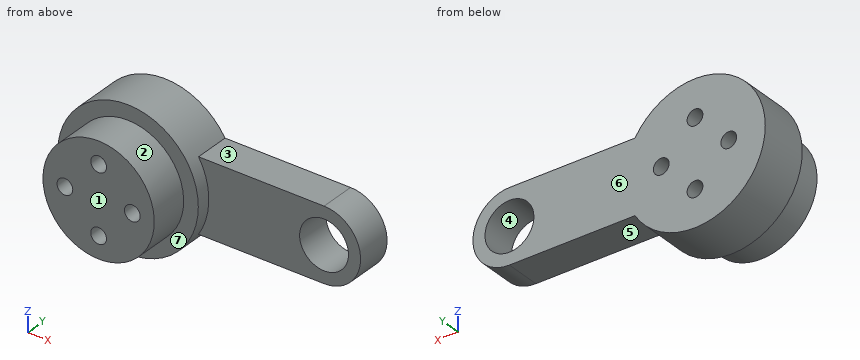
```python
from build123d import *

# Parameters (mm, degrees)
SKETCH_1_R      = 9.9
SKETCH_1_R_2    = 1.4
EXTRUDE_1_DEPTH = 7
SKETCH_2_R      = 12.5
SKETCH_2_R_2    = 1.4
EXTRUDE_2_DEPTH = 2.5
SKETCH_3_R      = 1.4
SKETCH_3_R_2    = 4.35
EXTRUDE_3_DEPTH = 6.3


with BuildPart() as part:
    # 草图1 → 凸台-拉伸1 (new body)
    with BuildSketch(Plane(origin=(0, 0, 0), x_dir=(1, 0, 0), z_dir=(0, 1, 0))):
        with Locations(Location((0, 0, 0), (0, 0, 270))):
            Circle(SKETCH_1_R)
        with Locations(Location((6, 0, 0), (0, 0, 270))):
            Circle(SKETCH_1_R_2, mode=Mode.SUBTRACT)
        with Locations(Location((0, -6, 0), (0, 0, 270))):
            Circle(SKETCH_1_R_2, mode=Mode.SUBTRACT)
        with Locations(Location((-6, 0, 0), (0, 0, 270))):
            Circle(SKETCH_1_R_2, mode=Mode.SUBTRACT)
        with Locations(Location((0, 6, 0), (0, 0, 270))):
            Circle(SKETCH_1_R_2, mode=Mode.SUBTRACT)
    extrude(amount=EXTRUDE_1_DEPTH)

    # 草图2 → 凸台-拉伸2 (add)
    with BuildSketch(Plane(origin=(0, 7, 0), x_dir=(1, 0, 0), z_dir=(0, 1, 0))):
        with Locations(Location((0, 0, 0), (0, 0, 270))):
            Circle(SKETCH_2_R)
        with Locations(Location((-6, 0, 0), (0, 0, 270))):
            Circle(SKETCH_2_R_2, mode=Mode.SUBTRACT)
        with Locations(Location((0, -6, 0), (0, 0, 270))):
            Circle(SKETCH_2_R_2, mode=Mode.SUBTRACT)
        with Locations(Location((6, 0, 0), (0, 0, 270))):
            Circle(SKETCH_2_R_2, mode=Mode.SUBTRACT)
        with Locations(Location((0, 6, 0), (0, 0, 270))):
            Circle(SKETCH_2_R_2, mode=Mode.SUBTRACT)
    extrude(amount=EXTRUDE_2_DEPTH)

    # 草图3 → 凸台-拉伸3 (add)
    with BuildSketch(Plane(origin=(0, 9.5, 0), x_dir=(1, 0, 0), z_dir=(0, 1, 0))):
        with BuildLine():
            Line((33, 6.5), (10.677078252, 6.5))
            ThreePointArc((10.677078252, 6.5), (-12.5, 0), (10.677078252, -6.5))
            Line((10.677078252, -6.5), (33, -6.5))
            ThreePointArc((33, -6.5), (39.5, 0), (33, 6.5))
        make_face()
        with Locations(Location((6, 0, 0), (0, 0, 270))):
            Circle(SKETCH_3_R, mode=Mode.SUBTRACT)
        with Locations(Location((-6, 0, 0), (0, 0, 270))):
            Circle(SKETCH_3_R, mode=Mode.SUBTRACT)
        with Locations(Location((33, 0, 0), (0, 0, 270))):
            Circle(SKETCH_3_R_2, mode=Mode.SUBTRACT)
        with Locations(Location((0, 6, 0), (0, 0, 270))):
            Circle(SKETCH_3_R, mode=Mode.SUBTRACT)
        with Locations(Location((0, -6, 0), (0, 0, 270))):
            Circle(SKETCH_3_R, mode=Mode.SUBTRACT)
    extrude(amount=EXTRUDE_3_DEPTH)


solid = part.part
```
The listing builds one solid part. Answer for the finished solid, in the listing's coordinates (mm). Face numbers are marked on the shaded views. A direction names the side the tool comes from. Coordinates: 2 decimals unless noted, no trailing zeros. Write each loop counter-clockwise with the first axis right and the second up, starting at its lowest first coordinate (ties: lowest second). Pieces come first, ordered by that corner, then holes. Notation, with made-up numbers: (78, -27.75) - (83, -27.75) arc R9 cw to (83, -11.75) - close; hole circle Ø10 at (25.5, -6). An arc over 180 degrees is marked (long way). Return JSON: item names as keys, results as strings. Group by question number.
Q1. For a pull along Z with two mould halves and no side action, classify the marked faces 1, 2, 3 and 4 as +Z half, -Z half, draft (parallel to the pull), parting line (faces both ways), or undercut.
Q2. Find the intervals of material crossed by line 1 along X through (y, z) = (13, 0); line 2 along X through (y, z) = (14.75, 1); line 3 along X through (y, z) = (11.5, -6), in increasing order. Write a range as [from, to].
Q3. The part is cut by section D-D on x = 32. Write down the section's boundary in (y, z), and give its area (3 significant figures).
Q4. The part is cut by section A-A on z = 0. Write down the section's boundary in (x, y).
Q5. The part is cut by section B-B on y = 12.25. Write down the section's boundary in (x, z), and give its area (3 significant figures).
Q6. Flat-ended cylindrical pins translate along their axes: pin 1 Ø5 at (x, y) = (24, 13.5) entering from -Z; pin 2 Ø1 at (y, z) = (7, 5) entering from +X; pin 3 Ø7 at (x, y) = (20.5, 13) entering from +Z. Find the tip coordinate at first contact, or state that the pin passes through.
Q7. The part is cut by section C-C on y = 7.75. Write down the section's boundary in (x, z).
Q8. Which of the six approach directions +Z, -Z, +X, -X, +Y, -Y give full straight-line access (tool end or side, diameter ignored) to the marked faces 5, 6 and 7?
Evaluation:
{
 "1": {"face 1": "draft", "face 2": "parting line", "face 3": "+Z half", "face 4": "undercut"},
 "2": {"line 1": "x = [-12.5, -7.4], [-4.6, 4.6], [7.4, 28.65], [37.35, 39.5]", "line 2": "x = [-12.46, -6.98], [-5.02, 5.02], [6.98, 28.77], [37.23, 39.42]", "line 3": "x = [-10.97, -1.4], [1.4, 35.5]"},
 "3": {"outline": "(9.5, -6.5) - (15.8, -6.5) - (15.8, -4.23) - (9.5, -4.23) - close; (9.5, 4.23) - (15.8, 4.23) - (15.8, 6.5) - (9.5, 6.5) - close", "area": "28.6 mm2"},
 "4": {"outline": "(-12.5, 7) - (-9.9, 7) - (-9.9, 0) - (-7.4, 0) - (-7.4, 15.8) - (-12.5, 15.8) - close; (-4.6, 0) - (4.6, 0) - (4.6, 15.8) - (-4.6, 15.8) - close; (7.4, 0) - (9.9, 0) - (9.9, 7) - (12.5, 7) - (12.5, 9.5) - (28.65, 9.5) - (28.65, 15.8) - (7.4, 15.8) - close; (37.35, 9.5) - (39.5, 9.5) - (39.5, 15.8) - (37.35, 15.8) - close"},
 "5": {"outline": "(10.68, -6.5) - (33, -6.5) arc R6.5 ccw to (33, 6.5) - (10.68, 6.5) arc R12.5 ccw (long way) to start; hole circle Ø2.8 at (-6, 0); hole circle Ø2.8 at (0, -6); hole circle Ø2.8 at (0, 6); hole circle Ø2.8 at (6, 0); hole circle Ø8.7 at (33, 0)", "area": "747 mm2"},
 "6": {"pin 1": "stops at z = -6.5", "pin 2": "stops at x = 11.66", "pin 3": "stops at z = 6.5"},
 "7": {"outline": "circle Ø25 at (0, 0); hole circle Ø2.8 at (-6, 0); hole circle Ø2.8 at (0, -6); hole circle Ø2.8 at (0, 6); hole circle Ø2.8 at (6, 0)"},
 "8": {"face 5": "-Z, +X, +Y, -Y", "face 6": "+Z, -Z, +X, -X, +Y", "face 7": "-Y"}
}
